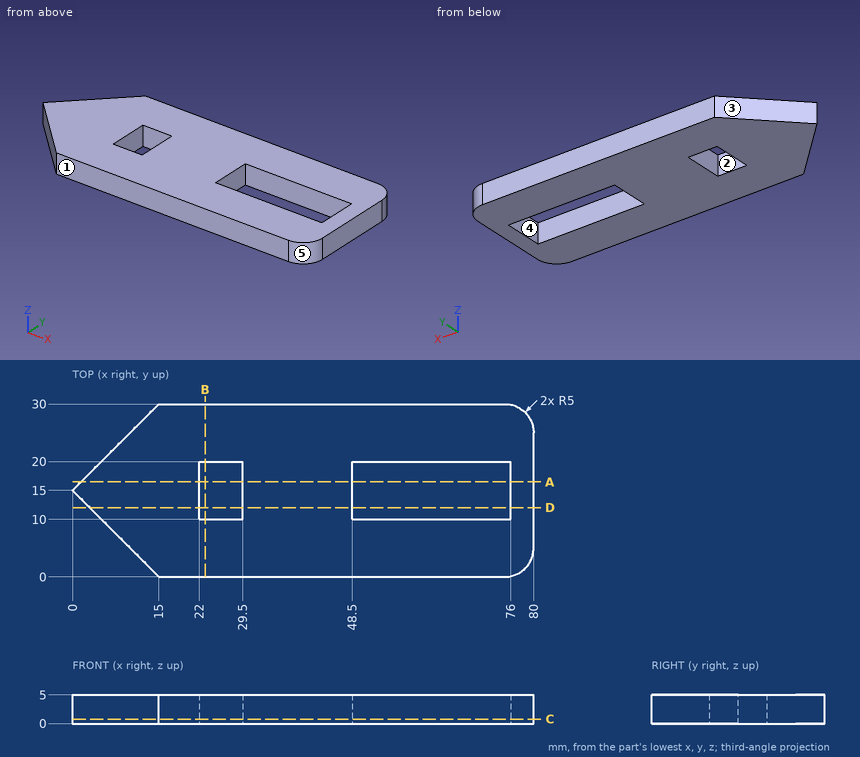
Here's the drawing with two shaded views (mm, measured from the low corner). I have some questions. A direction names the side the tool comes from. Coordinates: 2 decimals unless noted, no trailing zeros. Write each loop counter-clockwise with the first axis right and the second up, starting at its lowest first coordinate (ties: lowest second). Pieces come first, ordered by that corner, then holes.
Item 1: I want a section at D-D on y = 12. Write out the boundary of the cut face in (x, z), and give its area (3 significant figures).
Item 2: If we mould it in two halves opening along Y, with no side actions, what happens to the marked faces 3, 4 and 5? For each: +Y half, -Y half, draft (parallel to the pull), parting line (faces both ways), or undercut.
Item 3: I want a section at C-C on z = 0.8. Count the separate pieces of the cut face and the enclosed holes in it, and give its area (3 significant figures).
Item 4: If I drill on line 1 (Y direction, x = 74.5, z = 1.8); line 2 (X direction, y = 14, z = 0.95); line 3 (X direction, y = 16.5, z = 1.7), over which ranges is the centre line in solid material (lowest first)?
Item 5: I want a section at A-A on y = 16.5. Write out the boundary of the cut face in (x, z).
Item 6: Will these pins go through, and if not, where does the flat tip stop? pin 1 (1.5 mm diameter, centred on y = 16.5, z = 2, fed in from -X); pin 2 (1.5 mm diameter, centred on x = 9.5, z = 3.5, fed in from -Y); pin 3 (12 mm diameter, centred on x = 19.5, y = 5.5, fed in from -Z); pin 4 (1 mm diameter, centred on x = 49.5, y = 19, fed in from +Z).
Item 7: On a 3-axis mill with a long thin cutter (end or side, diameter ignored), from which of +Z, -Z, +X, -X, +Y, -Y can I reach the whole of each face in a straight line? I mean the marked faces 1 and 2. Say none if no direction works.
Item 8: I want a section at B-B on x = 23. Write out the boundary of the cut face in (y, z), and give its area (3 significant figures).
Findings below:
1. outline: (3, 0) - (22, 0) - (22, 5) - (3, 5) - close; (29.5, 0) - (48.5, 0) - (48.5, 5) - (29.5, 5) - close; (76, 0) - (80, 0) - (80, 5) - (76, 5) - close
1. area: 210 mm2
2. face 3: +Y half
2. face 4: undercut
2. face 5: -Y half
3. separate pieces: 1
3. enclosed holes: 2
3. area: 1,810 mm2
4. line 1: y = 0 to 10, 20 to 30
4. line 2: x = 1 to 22, 29.5 to 48.5, 76 to 80
4. line 3: x = 1.5 to 22, 29.5 to 48.5, 76 to 80
5. outline: (1.5, 0) - (22, 0) - (22, 5) - (1.5, 5) - close; (29.5, 0) - (48.5, 0) - (48.5, 5) - (29.5, 5) - close; (76, 0) - (80, 0) - (80, 5) - (76, 5) - close
6. pin 1: stops at x = 0.75
6. pin 2: stops at y = 4.75
6. pin 3: stops at z = 0
6. pin 4: passes through
7. face 1: +Z, -Z, +X, -X, -Y
7. face 2: +Z, -Z
8. outline: (0, 0) - (10, 0) - (10, 5) - (0, 5) - close; (20, 0) - (30, 0) - (30, 5) - (20, 5) - close
8. area: 100 mm2
